```python
from build123d import *

# Parameters (mm, degrees)
SKETCH1_R               = 25
SKETCH1_R_2             = 9.5
BOSS_EXTRUDE1_DEPTH     = 2
SKETCH2_R               = 12.5
SKETCH2_R_2             = 9.5
BOSS_EXTRUDE2_DEPTH     = 20
SKETCH3_R               = 2
CUT_EXTRUDE1_DEPTH      = 25
CIRPATTERN1_COUNT       = 4
CUT_EXTRUDE2_DEPTH      = 42.641325627
CUT_EXTRUDE2_DEPTH_BACK = 42.641325627
SKETCH4_R               = 2


with BuildPart() as part:
    # Sketch1 → Boss-Extrude1 (new body)
    with BuildSketch(Plane(origin=(0, 0, 0), x_dir=(1, 0, 0), z_dir=(0, 1, 0))):
        with Locations(Location((0, 0, 0), (0, 0, 270))):
            Circle(SKETCH1_R)
        with Locations(Location((0, 0, 0), (0, 0, 270))):
            Circle(SKETCH1_R_2, mode=Mode.SUBTRACT)
    extrude(amount=BOSS_EXTRUDE1_DEPTH)

    # Sketch2 → Boss-Extrude2 (add)
    with BuildSketch(Plane(origin=(0, 2, 0), x_dir=(1, 0, 0), z_dir=(0, 1, 0))):
        with Locations(Location((0, 0, 0), (0, 0, 270))):
            Circle(SKETCH2_R)
        with Locations(Location((0, 0, 0), (0, 0, 270))):
            Circle(SKETCH2_R_2, mode=Mode.SUBTRACT)
    extrude(amount=BOSS_EXTRUDE2_DEPTH)

    # Sketch3 → Cut-Extrude1 (cut)
    with BuildSketch(Plane(origin=(0, 2, 0), x_dir=(1, 0, 0), z_dir=(0, 1, 0))):
        with Locations(Location((0, 20, 0), (0, 0, 270))):
            Circle(SKETCH3_R)
    cut_extrude1 = extrude(amount=-CUT_EXTRUDE1_DEPTH, mode=Mode.SUBTRACT)

    # CirPattern1: Cut-Extrude1 ×4 about axis
    cirpattern1_axis = Axis((0, 0, 0), (0, 1, 0))
    for i in range(1, CIRPATTERN1_COUNT):
        add(cut_extrude1.rotate(cirpattern1_axis, i * 360 / CIRPATTERN1_COUNT), mode=Mode.SUBTRACT)

    # Sketch4 → Cut-Extrude2 (cut, two sides: drawn at the far end of the back side and taken through both)
    with BuildSketch(Plane(origin=(0, 0, 0), x_dir=(0, 0, -1), z_dir=(1, 0, 0)).offset(-CUT_EXTRUDE2_DEPTH_BACK)):
        with Locations((0, 14.24552707)):
            Circle(SKETCH4_R)
    extrude(amount=CUT_EXTRUDE2_DEPTH + CUT_EXTRUDE2_DEPTH_BACK, mode=Mode.SUBTRACT)


solid = part.part
```
CAD build for the part. Positions are in the model's coordinates, mm. A direction names the side the tool comes from. Give positions to 0.01 mm unless a question says otherwise; leave off trailing zeros. Write each loop counter-clockwise with the first axis right and the second up, starting at its lowest first coordinate (ties: lowest second). Pieces come first, ordered by that corner, then holes. Notation, with made-up numbers: (34.25, -35) -> (46.25, -35) arc R13 ccw to (46.25, -18) -> close; hole circle Ø9 at (-6, 25.5). An arc over 180 degrees is marked (long way). Write each question's results on one line, items separated by ' | '.
1. Two-plate mould, pull along X, no slides. Class faces 1 (the flat face through (9.3, 22, 2.7)), 2 (the cylindrical face through (7.509, 0.986, 23.846)), 3 (the cylindrical face through (21.6, 1, -1.2)), 4 (the cylindrical face through (-9.274, 10.846, -2.059)): pulls with the +X half, pulls with the -X half, needs draft (parallel to the pull), parting line crosses it, or undercut.
Geometry check:
face 1: needs draft | face 2: parting line crosses it | face 3: undercut | face 4: undercut
2. Wall check: probe 1 along X at (y, z) = (20.5, -0.5); probe 2 along Y at (x, z) = (10.4, 0); probe 3 along X at (y, z) = (6.75, -2.5). Give the ranges that are in metal, low to high. Write a range as [from, to].
Geometry check:
probe 1: [-12.49, -9.49], [9.49, 12.49] | probe 2: [0, 12.25], [16.25, 22] | probe 3: [-12.25, -9.17], [9.17, 12.25]
3. Drop flat-ended pins along their axis: P1, Ø5, axis at y = 14.25, z = 0, coming from the -X side; P2, Ø6, axis at x = -4, y = 18, coming from the -Z side; P3, Ø6, axis at x = -13.5, y = 14, coming from the +Z side; P4, Ø3, axis at x = 14.5, y = 10, coming from the -Z side. Give the stop position or say it passes through.
Geometry check:
P1: x = -12.5 | P2: z = -12.46 | P3: z = 6.78 | P4: through
4. Cut at D-D, the plane x = 0. Write the cut outline in (y, z), then the cut area to 3 significant figures.
Geometry check:
outline: (0, -25) -> (2, -25) -> (2, -22) -> (0, -22) -> close; (0, -18) -> (2, -18) -> (2, -12.5) -> (22, -12.5) -> (22, -9.5) -> (0, -9.5) -> close; (0, 9.5) -> (22, 9.5) -> (22, 12.5) -> (2, 12.5) -> (2, 18) -> (0, 18) -> close; (0, 22) -> (2, 22) -> (2, 25) -> (0, 25) -> close | area: 166 mm²
5. Cut at C-C, the plane z = 0. Write the cut outline in (x, y), then the cut area to 3 significant figures.
Geometry check:
outline: (-25, 0) -> (-22, 0) -> (-22, 2) -> (-25, 2) -> close; (-18, 0) -> (-9.5, 0) -> (-9.5, 12.25) -> (-12.5, 12.25) -> (-12.5, 2) -> (-18, 2) -> close; (-12.5, 16.25) -> (-9.5, 16.25) -> (-9.5, 22) -> (-12.5, 22) -> close; (9.5, 0) -> (18, 0) -> (18, 2) -> (12.5, 2) -> (12.5, 12.25) -> (9.5, 12.25) -> close; (9.5, 16.25) -> (12.5, 16.25) -> (12.5, 22) -> (9.5, 22) -> close; (22, 0) -> (25, 0) -> (25, 2) -> (22, 2) -> close | area: 142 mm²
6. Which spindle directions (+Z, -Z, +X, -X, +Y, -Y) get a long thin tool onto all of the face, cutting with end or side? Do faces 5 (the cylindrical face through (-11.09, 11.86, 5.77)), 6 (the cylindrical face through (-1.2, 1, -21.6)). Say none if no direction does.
Geometry check:
face 5: +Y | face 6: +Y, -Y
7. Cut at B-B, the plane z = -20. Write the cut outline in (x, y).
Geometry check:
outline: (-15, 0) -> (-2, 0) -> (-2, 2) -> (-15, 2) -> close; (2, 0) -> (15, 0) -> (15, 2) -> (2, 2) -> close
8. Cut at A-A, the plane x = -20. Write the cut outline in (y, z).
Geometry check:
outline: (0, -15) -> (2, -15) -> (2, -2) -> (0, -2) -> close; (0, 2) -> (2, 2) -> (2, 15) -> (0, 15) -> close
